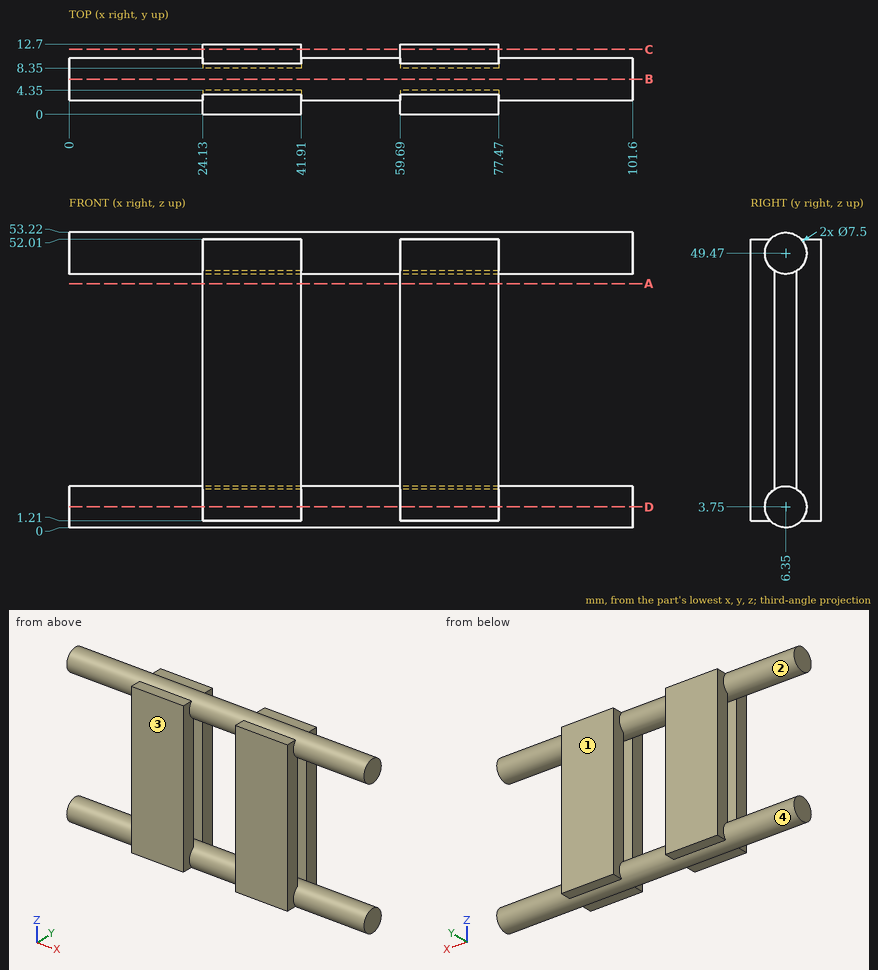
Design review of the part shown in the three views and the two pictorial views. Dimensions are in mm from the part's minimum x, y and z. A direction names the side the tool comes from. Round coordinates to 2 decimals unless told otherwise and drop trailing zeros. Write each loop counter-clockwise with the first axis right and the second up, starting at its lowest first coordinate (ties: lowest second). Pieces come first, ordered by that corner, then holes. Notation, with made-up numbers: (74.5, 26) - (119.5, 26) arc R28 ccw to (119.5, 60) - close; hole circle Ø9 at (22, 81). An arc over 180 degrees is marked (long way). Write item = value, one per line. Start each with the question number.
1. Draft analysis for pull direction Z (two halves, no side actions). For the marked faces 1 and 2, state which applies: released by +Z, released by -Z, zero draft, split by the parting line, or undercut.
2. Consider section A-A on z = 44. State the section outline as (x, y) points.
3. Consider section D-D on z = 3.75. State the section outline as (x, y) points.
4. Consider section B-B on y = 6.35. State the section outline as (x, z) points.
5. For the marked faces 3 and 4, list the 3-axis set-ups (+Z, -Z, +X, -X, +Y, -Y) from which the entire face can be reached by the end or side of a thin tool; tool diameter is ignored.
6. Consider section C-C on y = 11.75. State the section outline as (x, z) points.
7. For pin 1 Ø4 at (x, y) = (65, 3) entering from -Z; pin 2 Ø3 at (x, y) = (50.5, 11) entering from +Z; pin 3 Ø1.1 at (x, y) = (70, 10) entering from -Z; pin 4 Ø14 at (x, z) = (36.5, 19) entering from -Y, all flat-tipped, find the tip position at first contact; note any pin that passes through.
8. Wall thickness on L1, parallel to X at y = 11, z = 6; L2, parallel to Y at x = 77, z = 43; L3, parallel to Z at x = 87, y = 7.75: over which ranges is each line inside the solid? List them lowest first.
Evaluation:
q1.face_1 = zero draft
q1.face_2 = undercut
q2.outline = (24.13, 0) - (41.91, 0) - (41.91, 4.35) - (24.13, 4.35) - close; (24.13, 8.35) - (41.91, 8.35) - (41.91, 12.7) - (24.13, 12.7) - close; (59.69, 0) - (77.47, 0) - (77.47, 4.35) - (59.69, 4.35) - close; (59.69, 8.35) - (77.47, 8.35) - (77.47, 12.7) - (59.69, 12.7) - close
q3.outline = (0, 2.6) - (24.13, 2.6) - (24.13, 0) - (41.91, 0) - (41.91, 2.6) - (59.69, 2.6) - (59.69, 0) - (77.47, 0) - (77.47, 2.6) - (101.6, 2.6) - (101.6, 10.1) - (77.47, 10.1) - (77.47, 12.7) - (59.69, 12.7) - (59.69, 10.1) - (41.91, 10.1) - (41.91, 12.7) - (24.13, 12.7) - (24.13, 10.1) - (0, 10.1) - close
q4.outline = (0, 0) - (101.6, 0) - (101.6, 7.5) - (0, 7.5) - close; (0, 45.72) - (101.6, 45.72) - (101.6, 53.22) - (0, 53.22) - close
q5.face_3 = +Z, -Z, +X, -X, -Y
q5.face_4 = none
q6.outline = (24.13, 1.21) - (41.91, 1.21) - (41.91, 52.01) - (24.13, 52.01) - close; (59.69, 1.21) - (77.47, 1.21) - (77.47, 52.01) - (59.69, 52.01) - close
q7.pin_1 = 0.25
q7.pin_2 = 51.5
q7.pin_3 = 1.21
q7.pin_4 = 0
q8.L1 = 24.13 to 41.91, 59.69 to 77.47
q8.L2 = 0 to 4.35, 8.35 to 12.7
q8.L3 = 0.27 to 7.23, 45.99 to 52.95
